Source: CAD feature listing. Evaluate the final solid. Frame: model axes, mm. A direction names the side the tool comes from. Give positions to 0.01 mm unless a question says otherwise; leave off trailing zeros. Write each loop counter-clockwise with the first axis right and the second up, starting at its lowest first coordinate (ties: lowest second). Pieces come first, ordered by that corner, then holes. Notation, with made-up numbers: M 35.25,60.5 L 43.25,60.5 A24 cw 43.25,90.5 Z; hole C 2.25,89.25 d11. An arc over 180 degrees is marked long. Answer as a JSON object with one key per item and string values. Group by question number.
Autodesk Inventor part; units mm, degrees
ref_plane "YZ Plane" through (0, 0, 0) normal (1, 0, 0) x (0, 1, 0)
ref_plane "XZ Plane" through (0, 0, 0) normal (0, 1, 0) x (-1, 0, 0)
ref_plane "XY Plane" through (0, 0, 0) normal (0, 0, 1) x (1, 0, 0)
sketch "Sketch1" plane through (0, 0, 0) normal (0, 1, 0) x (-1, 0, 0)
  circle A0 centre (0, 0) radius 12.5
  dimension "d0" = 25
extrude "Extrusion1" add sketch "Sketch1" along normal blind 11
chamfer "Chamfer1" distance 7.5 distance2 11 1 edges at (12.5, 11, 0) measured on face at (-2.488, 11, -2.432)
sketch "Sketch2" plane through (0, 11, 0) normal (0, 1, 0) x (1, 0, 0)
  circle A0 centre (0, 0) radius 5
  circle A1 centre (0, 0) radius 5
extrude "Extrusion2" add sketch "Sketch2" along normal blind 9
sketch "Sketch3" plane through (0, 0, 0) normal (0, -1, 0) x (1, 0, 0)
  circle A0 centre (0, 0) radius 2.4
  dimension "d8" = 4.8
extrude "Extrusion3" add sketch "Sketch3" along normal blind 4.8
properties part number "pladsholder"
(1) Ray query, L1, parallel to Y at x = 4.5, z = -1.5; L2, parallel to X at y = 1.25, z = 10.5; L3, parallel to X at y = -2, z = -2. Return the intervals inside material, ascending. Write a range as [from, to].
(2) Section C-C, the plane y = -2.75. Return loops of the section in (x, z), plus the area to 3 significant figures.
(3) Contact query for flat-ended pins moving along their axis: pin 1 Ø1.5 at (x, z) = (-6, -5) entering from -Y; pin 2 Ø5 at (x, z) = (-6.5, -9.5) entering from +Y; pin 3 Ø4 at (x, y) = (-5, 2.5) entering from +Z. Output: stop coordinate, or through.
(4) Access query for faces 1 (the cylindrical face through (1.29, -2.366, -2.024)), 2 (the cylindrical face through (-1.08, 15.44, -4.88)), 3 (the flat face through (0, 20, 0)). Directions: +Z, -Z, +X, -X, +Y, -Y. A direction counts if a zero-diameter tool reaches every point of the face in a straight line with its end or side. Return the directions, or none.
(5) Section D-D, the plane y = 17.5. Return loops of the section in (x, z), plus the area to 3 significant figures.
Reported:
{
 "1": {"L1": "y = [0, 20]", "L2": "x = [-5.04, 5.04]", "L3": "x = [-1.33, 1.33]"},
 "2": {"outline": "C 0,0 d4.8", "area": "18.1 mm2"},
 "3": {"pin 1": "stops at y = 0", "pin 2": "stops at y = 5.12", "pin 3": "stops at z = 11.29"},
 "4": {"face 1": "-Y", "face 2": "+Y", "face 3": "+Z, -Z, +X, -X, +Y"},
 "5": {"outline": "C 0,0 d10", "area": "78.5 mm2"}
}
